from build123d import *

# Parameters (mm, degrees)
SKETCH1_W           = 66.26
SKETCH1_H           = 78.34
BOSS_EXTRUDE1_DEPTH = 1.55
SKETCH2_R           = 2.5
CUT_EXTRUDE1_DEPTH  = 16.55
SKETCH3_R           = 2.5
CUT_EXTRUDE2_DEPTH  = 16.55
SKETCH4_W           = 6.76
SKETCH4_H           = 67.34
BOSS_EXTRUDE2_DEPTH = 9.18
SKETCH7_W           = 10.2328791
SKETCH7_H           = 9.710793432
BOSS_EXTRUDE3_DEPTH = 15.86


with BuildPart() as part:
    # Sketch1 → Boss-Extrude1 (new body)
    with BuildSketch(Plane.XY):
        Rectangle(SKETCH1_W, SKETCH1_H)
    extrude(amount=BOSS_EXTRUDE1_DEPTH)

    # Sketch2 → Cut-Extrude1 (cut)
    with BuildSketch(Plane.XY.offset(1.55)):
        with Locations((-30.076432851, 36.090160922)):
            Circle(SKETCH2_R)
    cut_extrude1 = extrude(amount=-CUT_EXTRUDE1_DEPTH, mode=Mode.SUBTRACT)

    # Sketch3 → Cut-Extrude2 (cut)
    with BuildSketch(Plane.XY.offset(1.55)):
        with Locations((-30.076432851, -36.07)):
            Circle(SKETCH3_R)
    cut_extrude2 = extrude(amount=-CUT_EXTRUDE2_DEPTH, mode=Mode.SUBTRACT)

    # Mirror1: Cut-Extrude1, Cut-Extrude2 across plane
    add(cut_extrude1.mirror(Plane(origin=(0, 0, 0), x_dir=(0, 0, 1), z_dir=(1, 0, 0))), mode=Mode.SUBTRACT)
    add(cut_extrude2.mirror(Plane(origin=(0, 0, 0), x_dir=(0, 0, 1), z_dir=(1, 0, 0))), mode=Mode.SUBTRACT)

    # Sketch4 → Boss-Extrude2 (add)
    with BuildSketch(Plane.XY.offset(1.55)):
        with Locations((-24.196432851, -0.24)):
            Rectangle(SKETCH4_W, SKETCH4_H)
    boss_extrude2 = extrude(amount=BOSS_EXTRUDE2_DEPTH)

    # Mirror2: Boss-Extrude2 across plane
    add(boss_extrude2.mirror(Plane(origin=(0, 0, 0), x_dir=(0, 0, 1), z_dir=(1, 0, 0))))

    # Sketch7 → Boss-Extrude3 (add)
    with BuildSketch(Plane.XY.offset(1.55)):
        Rectangle(SKETCH7_W, SKETCH7_H)
    extrude(amount=BOSS_EXTRUDE3_DEPTH)


solid = part.part
Part model, mm, in its own coordinate system. A direction names the side the tool comes from. Coordinates: 2 decimals unless noted, no trailing zeros. Loops run counter-clockwise (first coordinate to the right, second up) from the corner with the lowest first, then second, coordinate; pieces in that order, holes last. Notation, with made-up numbers: (-8, 27.5) -> (11, 27.5) arc R23 cw to (11, 57.5) -> close; hole circle Ø9 at (42.25, 54.25). An arc over 180 degrees is marked (long way). Use a Markdown table: item, result. Add a question column.
Item 1: Band-saw the part on B-B on z = 8.25. Write the cut outline in (x, y), plus the area to 3 significant figures.
Item 2: Flat gauge pins, fed straight in: P1, Ø3, axis at y = 10, z = 8.5, coming from the +X side; P2, Ø3, axis at y = -0.5, z = 7, coming from the -X side; P3, Ø6.5, axis at x = 30.08, y = 36.09, coming from the +Z side; P4, Ø4, axis at x = -30.08, y = -36.07, coming from the -Z side. Where does each tip first touch, or does it go through?
Item 3: Pull direction X, two halves, no side cores. Call faces 4 (the cylindrical face through (-30.62, -38.51, 0.79)), 5 (the flat face through (-24, -33.91, 6)), 6 (the flat face through (27.576, -1, 6)): +X half, -X half, draft (parallel to the pull), parting line (faces both ways), or undercut.
Item 4: Which spindle directions (+Z, -Z, +X, -X, +Y, -Y) get a long thin tool onto all of the face, cutting with end or side? Do faces 1 (the flat face through (24, -33.91, 6)), 2 (the flat face through (24, 33.43, 6)), 3 (the flat face through (-20.816, -1, 6)). Say none if no direction does.
Item 5: Band-saw the part on C-C on x = -24. Write the cut outline in (y, z).
Item 6: Band-saw the part on D-D on y = -1.5. Write the cut outline in (x, z).
Item 7: Probe probe 1 along X at (y, z) = (-2.5, 9.75); probe 2 along X at (y, z) = (-19.5, 10); probe 3 along Y at (x, z) = (1.5, 10.5). List the from-to ranges inside material, lowest first.
Item 8: Band-saw the part on A-A on y = -36.07. Write the cut outline in (x, z).
Geometry says:
| question | item | result |
|---|---|---|
| 1 | outline | (-27.58, -33.91) -> (-20.82, -33.91) -> (-20.82, 33.43) -> (-27.58, 33.43) -> close; (-5.12, -4.86) -> (5.12, -4.86) -> (5.12, 4.86) -> (-5.12, 4.86) -> close; (20.82, -33.91) -> (27.58, -33.91) -> (27.58, 33.43) -> (20.82, 33.43) -> close |
| 1 | area | 1,010 mm² |
| 2 | P1 | x = 27.58 |
| 2 | P2 | x = -27.58 |
| 2 | P3 | z = 1.55 |
| 2 | P4 | through |
| 3 | face 4 | undercut |
| 3 | face 5 | draft |
| 3 | face 6 | +X half |
| 4 | face 1 | +Z, +X, -X, -Y |
| 4 | face 2 | +Z, +X, -X, +Y |
| 4 | face 3 | +Z, +Y, -Y |
| 5 | outline | (-39.17, 0) -> (39.17, 0) -> (39.17, 1.55) -> (33.43, 1.55) -> (33.43, 10.73) -> (-33.91, 10.73) -> (-33.91, 1.55) -> (-39.17, 1.55) -> close |
| 6 | outline | (-33.13, 0) -> (33.13, 0) -> (33.13, 1.55) -> (27.58, 1.55) -> (27.58, 10.73) -> (20.82, 10.73) -> (20.82, 1.55) -> (5.12, 1.55) -> (5.12, 17.41) -> (-5.12, 17.41) -> (-5.12, 1.55) -> (-20.82, 1.55) -> (-20.82, 10.73) -> (-27.58, 10.73) -> (-27.58, 1.55) -> (-33.13, 1.55) -> close |
| 7 | probe 1 | -27.58 to -20.82, -5.12 to 5.12, 20.82 to 27.58 |
| 7 | probe 2 | -27.58 to -20.82, 20.82 to 27.58 |
| 7 | probe 3 | -4.86 to 4.86 |
| 8 | outline | (-33.13, 0) -> (-32.58, 0) -> (-32.58, 1.55) -> (-33.13, 1.55) -> close; (-27.58, 0) -> (27.58, 0) -> (27.58, 1.55) -> (-27.58, 1.55) -> close; (32.58, 0) -> (33.13, 0) -> (33.13, 1.55) -> (32.58, 1.55) -> close |
